Here's how the part is built. I have some questions about the finished solid (model axes, mm). A direction names the side the tool comes from. Give positions to 0.01 mm unless a question says otherwise; leave off trailing zeros. Order: outer loops, then holes, each group sorted by start corner. A loop starts at its lowest first (then second) coordinate and runs counter-clockwise, first axis right, second up.
from build123d import *

# Parameters (mm, degrees)
SKETCH1_W                      = 138
SKETCH1_H                      = 50
BOSS_EXTRUDE1_DEPTH            = 62
SKETCH2_W                      = 82
SKETCH2_H                      = 8
CUT_EXTRUDE1_DEPTH             = 160.336122709
SKETCH3_W                      = 56
SKETCH3_H                      = 62
CUT_EXTRUDE2_DEPTH             = 23
CUT_EXTRUDE3_DEPTH             = 19
SKETCH5_W                      = 36
SKETCH5_H                      = 15
CUT_EXTRUDE4_DEPTH             = 157.396930916
M3X0_5_TAPPED_HOLE1_D          = 2.5
M3X0_5_TAPPED_HOLE1_DEPTH      = 12.4
M3X0_5_TAPPED_HOLE1_TIP        = 0.751075774
M4X0_7_TAPPED_HOLE1_D          = 3.3
M4X0_7_TAPPED_HOLE1_DEPTH      = 10.1
M4X0_7_TAPPED_HOLE1_TIP        = 0.991420021
F_3_1_3_1_DIAMETER_HOLE1_D     = 3.1
F_3_1_3_1_DIAMETER_HOLE1_DEPTH = 10
F_3_1_3_1_DIAMETER_HOLE1_TIP   = 0.931333959
SKETCH15_W                     = 82
SKETCH15_H                     = 2.7
CUT_EXTRUDE6_DEPTH             = 160.336122709
SKETCH16_W                     = 8.5
SKETCH16_H                     = 24
CUT_EXTRUDE7_DEPTH             = 5
M3X0_5_TAPPED_HOLE2_D          = 2.5
M3X0_5_TAPPED_HOLE2_DEPTH      = 7.5
M3X0_5_TAPPED_HOLE2_TIP        = 0.751075774
M5X0_8_TAPPED_HOLE1_D          = 4.2
M5X0_8_TAPPED_HOLE1_DEPTH      = 12.4
M5X0_8_TAPPED_HOLE1_TIP        = 1.2618073


with BuildPart() as part:
    # Sketch1 → Boss-Extrude1 (new body)
    with BuildSketch(Plane(origin=(0, 0, 0), x_dir=(1, 0, 0), z_dir=(0, 1, 0))):
        with Locations((69, 25)):
            Rectangle(SKETCH1_W, SKETCH1_H)
    extrude(amount=-BOSS_EXTRUDE1_DEPTH)

    # Sketch2 → Cut-Extrude1 (cut, through all)
    with BuildSketch(Plane.XY):
        with Locations((41, -4)):
            Rectangle(SKETCH2_W, SKETCH2_H)
    extrude(amount=-CUT_EXTRUDE1_DEPTH, mode=Mode.SUBTRACT)

    # Sketch3 → Cut-Extrude2 (cut)
    with BuildSketch(Plane.XY):
        with Locations((110, -31)):
            Rectangle(SKETCH3_W, SKETCH3_H)
    extrude(amount=-CUT_EXTRUDE2_DEPTH, mode=Mode.SUBTRACT)

    # Sketch4 → Cut-Extrude3 (cut)
    with BuildSketch(Plane(origin=(0, -8, 0), x_dir=(1, 0, 0), z_dir=(0, 1, 0))):
        Polygon((40, 36.5), (54.1, 36.5), (54.1, 0), (43, 0), (43, 20.5), (40, 20.5), align=None)
    extrude(amount=-CUT_EXTRUDE3_DEPTH, mode=Mode.SUBTRACT)

    # Sketch5 → Cut-Extrude4 (cut, through all)
    with BuildSketch(Plane(origin=(0, -8, 0), x_dir=(1, 0, 0), z_dir=(0, 1, 0))):
        with Locations((64, 7.5)):
            Rectangle(SKETCH5_W, SKETCH5_H)
    extrude(amount=-CUT_EXTRUDE4_DEPTH, mode=Mode.SUBTRACT)

    # M3x0.5 Tapped Hole1
    with Locations(Plane.XY):
        with Locations((5, -15), (35, -25)):
            Hole(M3X0_5_TAPPED_HOLE1_D / 2, depth=M3X0_5_TAPPED_HOLE1_DEPTH)
            with Locations((0, 0, -(M3X0_5_TAPPED_HOLE1_DEPTH + M3X0_5_TAPPED_HOLE1_TIP / 2))):  # 118° drill point
                Cone(0, M3X0_5_TAPPED_HOLE1_D / 2, M3X0_5_TAPPED_HOLE1_TIP, mode=Mode.SUBTRACT)

    # M4x0.7 Tapped Hole1
    with Locations(Plane(origin=(0, -62, 0), x_dir=(-1, 0, 0), z_dir=(0, -1, 0))):
        with Locations((-128, 35), (-10, 35)):
            Hole(M4X0_7_TAPPED_HOLE1_D / 2, depth=M4X0_7_TAPPED_HOLE1_DEPTH)
            with Locations((0, 0, -(M4X0_7_TAPPED_HOLE1_DEPTH + M4X0_7_TAPPED_HOLE1_TIP / 2))):  # 118° drill point
                Cone(0, M4X0_7_TAPPED_HOLE1_D / 2, M4X0_7_TAPPED_HOLE1_TIP, mode=Mode.SUBTRACT)

    # Ø3.1 (3.1) Diameter Hole1
    with Locations(Plane(origin=(46, 0, 0), x_dir=(0, 0, -1), z_dir=(1, 0, 0))):
        with Locations((4, -31), (12, -31)):
            Hole(F_3_1_3_1_DIAMETER_HOLE1_D / 2, depth=F_3_1_3_1_DIAMETER_HOLE1_DEPTH)
            with Locations((0, 0, -(F_3_1_3_1_DIAMETER_HOLE1_DEPTH + F_3_1_3_1_DIAMETER_HOLE1_TIP / 2))):  # 118° drill point
                Cone(0, F_3_1_3_1_DIAMETER_HOLE1_D / 2, F_3_1_3_1_DIAMETER_HOLE1_TIP, mode=Mode.SUBTRACT)

    # Sketch15 → Cut-Extrude6 (cut, through all)
    with BuildSketch(Plane.XY):
        with Locations((41, -9.35)):
            Rectangle(SKETCH15_W, SKETCH15_H)
    extrude(amount=-CUT_EXTRUDE6_DEPTH, mode=Mode.SUBTRACT)

    # Sketch16 → Cut-Extrude7 (cut)
    with BuildSketch(Plane(origin=(0, -10.7, 0), x_dir=(1, 0, 0), z_dir=(0, 1, 0))):
        with Locations((62.75, 38)):
            Rectangle(SKETCH16_W, SKETCH16_H)
    extrude(amount=-CUT_EXTRUDE7_DEPTH, mode=Mode.SUBTRACT)

    # M3x0.5 Tapped Hole2
    with Locations(Plane(origin=(0, -15.7, 0), x_dir=(1, 0, 0), z_dir=(0, 1, 0))):
        with Locations((62.75, 44)):
            Hole(M3X0_5_TAPPED_HOLE2_D / 2, depth=M3X0_5_TAPPED_HOLE2_DEPTH)
            with Locations((0, 0, -(M3X0_5_TAPPED_HOLE2_DEPTH + M3X0_5_TAPPED_HOLE2_TIP / 2))):  # 118° drill point
                Cone(0, M3X0_5_TAPPED_HOLE2_D / 2, M3X0_5_TAPPED_HOLE2_TIP, mode=Mode.SUBTRACT)

    # M5x0.8 Tapped Hole1
    with Locations(Plane.XY.offset(-23)):
        with Locations((88, -7), (88, -31)):
            Hole(M5X0_8_TAPPED_HOLE1_D / 2, depth=M5X0_8_TAPPED_HOLE1_DEPTH)
            with Locations((0, 0, -(M5X0_8_TAPPED_HOLE1_DEPTH + M5X0_8_TAPPED_HOLE1_TIP / 2))):  # 118° drill point
                Cone(0, M5X0_8_TAPPED_HOLE1_D / 2, M5X0_8_TAPPED_HOLE1_TIP, mode=Mode.SUBTRACT)


solid = part.part
Q1. If we section it at A-A on y = -21.5: List the corners of the cut face in (x, z) for me, plus the area to 3 significant figures.
Filled sheet:
outline: (0, -50) - (138, -50) - (138, -23) - (82, -23) - (82, -15) - (54.1, -15) - (54.1, -36.5) - (40, -36.5) - (40, -20.5) - (43, -20.5) - (43, 0) - (0, 0) - close; hole circle Ø2.5 at (62.75, -44)
area: 4,740 mm2
Q2. I need wall thicknesses on L1, parallel to X at y = -13.5, z = -28.5; L2, parallel to X at y = -25, z = -6.5; L3, parallel to Z at x = 128, y = -54. Which ranges of each line are inside material? Lowest first, please.
Filled sheet:
L1: x = 0 to 40, 54.1 to 58.5, 67 to 138
L2: x = 0 to 33.75, 36.25 to 43
L3: z = -50 to -36.65, -33.35 to -23
Q3. If we section it at B-B on x = 41.5: List the corners of the cut face in (y, z) for me, plus the area to 3 significant figures.
Filled sheet:
outline: (-62, -50) - (-10.7, -50) - (-10.7, -36.5) - (-27, -36.5) - (-27, -20.5) - (-10.7, -20.5) - (-10.7, 0) - (-62, 0) - close; hole circle Ø3.1 at (-31, -12); hole circle Ø3.1 at (-31, -4)
area: 2,290 mm2
Q4. If we section it at D-D on x = 92: List the corners of the cut face in (y, z) for me.
Filled sheet:
outline: (-62, -50) - (0, -50) - (0, -23) - (-62, -23) - close
Q5. Thinking about a two-plate mould opening in Z: for faces 5 (the face through (46, -44, -7)), 6 (the face through (88.2, -30.69, -36.44)), 7 (the face through (42, -19, -20.5)), 8 (the face through (9.9, -51.1, -34.7)), which applies, released by +Z, released by -Z, zero draft, split by the parting line, or undercut?
Filled sheet:
face 5: zero draft
face 6: released by +Z
face 7: undercut
face 8: undercut
Q6. I'm going to push flat-ended pins straight in: P1, Ø17, axis at x = 104, y = -45.5, coming from the +Z side; P2, Ø2.5, axis at x = 61.5, z = -38.5, coming from the +Y side; P3, Ø15.5, axis at x = 45.5, z = -17, coming from the +Y side. Where does each tip first touch, or does it pass through?
Filled sheet:
P1: stops at z = -23
P2: stops at y = -15.7
P3: stops at y = -10.7
Q7. If we section it at C-C on x = 78: List the corners of the cut face in (y, z) for me, plus the area to 3 significant figures.
Filled sheet:
outline: (-62, -50) - (-10.7, -50) - (-10.7, -15) - (-62, -15) - close
area: 1,800 mm2
Q8. For faces 1 (the face through (63, -13, -26)), 2 (the face through (82, -5, -36)), 3 (the face through (61.56, -19.5, -44.38)), 4 (the face through (90.1, -6.91, -29.29)), which set-ups out of +Z, -Z, +X, -X, +Y, -Y let a thin tool reach every point of the face, with its end or its side?
Filled sheet:
face 1: -Z, +Y
face 2: +Z, -Z, -X, +Y
face 3: +Y
face 4: +Z
